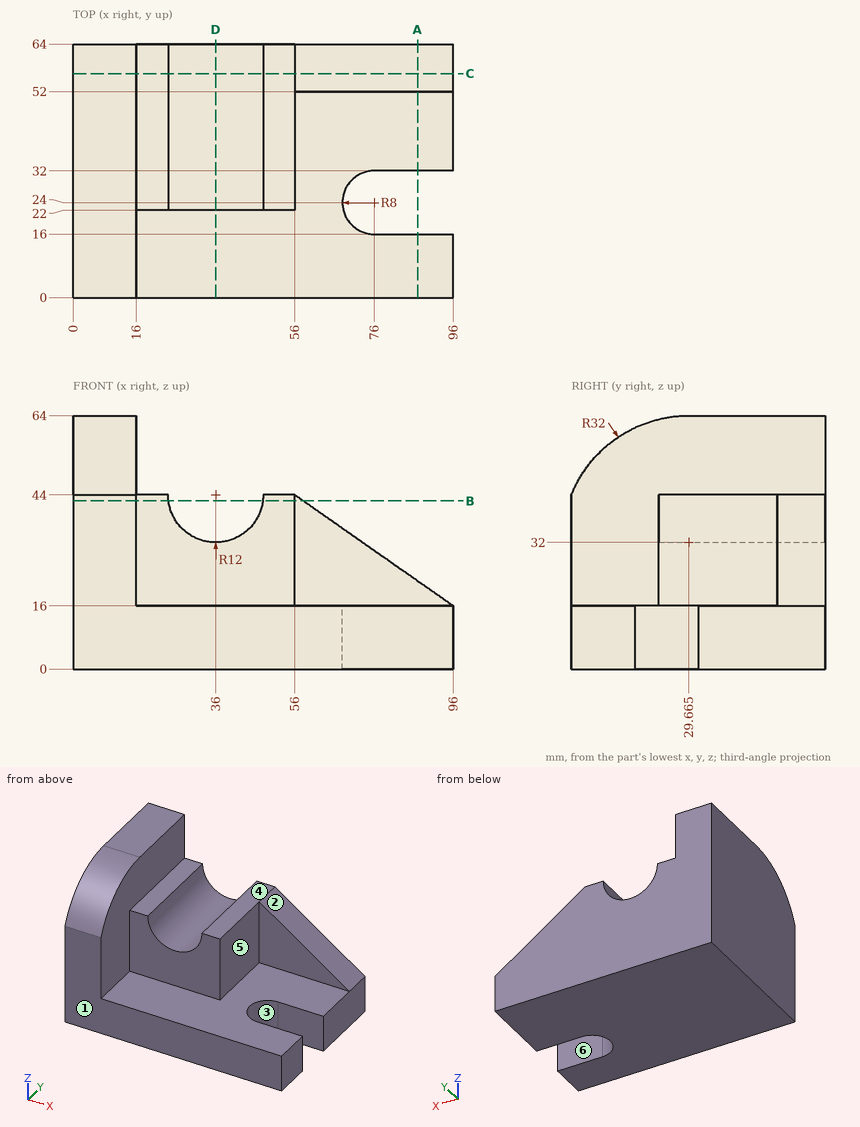
Verification items for this drawing (mm, ordinates from the low corner). A direction names the side the tool comes from. Round coordinates to 2 decimals unless told otherwise and drop trailing zeros. Order: outer loops, then holes, each group sorted by start corner. A loop starts at its lowest first (then second) coordinate and runs counter-clockwise, first axis right, second up. Notation, with made-up numbers: (-11.75, 66.5) - (6.25, 66.5) arc R17 cw to (6.25, 73.5) - close; hole circle Ø1 at (69, 12). An arc over 180 degrees is marked (long way). Answer as CSV lines item,"result". Start each with the question number.
1) Draft check along Y on the marked faces 1, 2 and 3. Enter one of: +Y half, -Y half, draft (parallel to the pull), parting line (faces both ways), or undercut.
2) Scan lines: probe 1 along Z at (x, y) = (77, 35); probe 2 along Y at (x, z) = (51, 28.5); probe 3 along Z at (x, y) = (36.5, 39). Record each from-to range of solid material in increasing order.
3) Section check B-B (z = 42.5). Record the cut outline in (x, y).
4) Section check D-D (x = 36). Record the cut outline in (y, z).
5) Section check C-C (y = 56.5). Record the cut outline in (x, z).
6) Section check A-A (x = 87). Record the cut outline in (y, z).
7) Tool access check on the marked faces 4, 5 and 6. Record the directions out of +Z, -Z, +X, -X, +Y, -Y that give a thin tool (end or side, any length) a straight path to the whole face; none if there is none.
8) Depth check by flat-ended pin: pin 1 (6 mm diameter, centred on x = 59.5, y = 38.5, fed in from +Z); pin 2 (14 mm diameter, centred on x = 46, z = 36.5, fed in from -Y); pin 3 (1.5 mm diameter, centred on y = 38, z = 17, fed in from +X). Enter the tip coordinate at first touch or a pass-through.
Determined:
1,face 1,"-Y half"
1,face 2,"draft"
1,face 3,"undercut"
2,probe 1,"0 to 16"
2,probe 2,"22 to 64"
2,probe 3,"0 to 32.01"
3,outline,"(0, 0) - (16, 0) - (16, 22) - (24.09, 22) - (24.09, 64) - (0, 64) - close; (47.91, 22) - (56, 22) - (56, 52) - (58.14, 52) - (58.14, 64) - (47.91, 64) - close"
4,outline,"(0, 0) - (64, 0) - (64, 32) - (22, 32) - (22, 16) - (0, 16) - close"
5,outline,"(0, 0) - (96, 0) - (96, 16) - (56, 44) - (48, 44) arc R12 cw to (24, 44) - (16, 44) - (16, 64) - (0, 64) - close"
6,outline,"(0, 0) - (16, 0) - (16, 16) - (0, 16) - close; (32, 0) - (64, 0) - (64, 22.3) - (52, 22.3) - (52, 16) - (32, 16) - close"
7,face 4,"+Z, +X, +Y, -Y"
7,face 5,"+Z, +X, -Y"
7,face 6,"+Z, -Z, +X"
8,pin 1,"z = 16"
8,pin 2,"y = 22"
8,pin 3,"x = 56"
